Geometry check sheet. Reference: the model listing, model coordinates, mm. Face numbers are marked on the shaded views. A direction names the side the tool comes from. Coordinates: 2 decimals unless noted, no trailing zeros. Write each loop counter-clockwise with the first axis right and the second up, starting at its lowest first coordinate (ties: lowest second). Pieces come first, ordered by that corner, then holes. Notation, with made-up numbers: (20.5, -30.5) -> (40.5, -30.5) arc R13 ccw to (40.5, -15.5) -> close; hole circle Ø6 at (-2.75, -34.5). An arc over 180 degrees is marked (long way). Answer in a Markdown table with one row per item. Add a question column.
1. Depth check by flat-ended pin: P1, Ø20.5, axis at y = -92.5, z = -40, coming from the +X side; P2, Ø10, axis at y = 48.5, z = 3.5, coming from the +X side; P3, Ø4, axis at x = -20.5, z = -41, coming from the +Y side. Enter the tip coordinate at first touch or a pass-through.
2. Cross-section at D-D on y = -37. Record the cut outline in (x, z).
3. Set-up check for the marked faces 1, 2, 3, 4 and 5: record each of +Z, -Z, +X, -X, +Y, -Y from which the full face is reachable in a straight line by a thin tool's end or side.
4. Cross-section at A-A on y = 65.5. Record the cut outline in (x, z).
5. Cross-section at B-B on z = -23. Record the cut outline in (x, y).
6. Scan lines: L1, parallel to Y at x = 13.5, z = -5; L2, parallel to Z at x = 7, y = 29.5; L3, parallel to Z at x = 75.5, y = 95. Record each from-to range of solid material in increasing order. Write a range as from..to.
7. Cross-section at C-C on x = -9. Record the cut outline in (y, z), and give its area (3 significant figures).
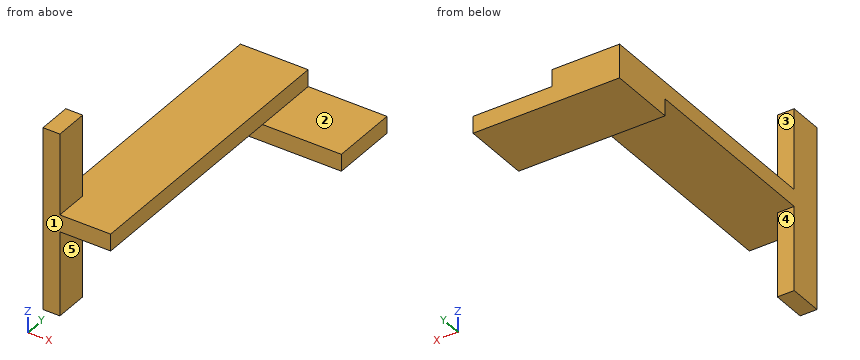
```python
from build123d import *

# Parameters (mm, degrees)
CROQUIS1_W              = 50.8
CROQUIS1_H              = 220
SALIENTE_EXTRUIR1_DEPTH = 12.7
CROQUIS2_W              = 110
CROQUIS2_H              = 50.8
SALIENTE_EXTRUIR2_DEPTH = 12.7
CROQUIS3_W              = 136.757374057
CROQUIS3_H              = 25.4
SALIENTE_EXTRUIR3_DEPTH = 12.7


with BuildPart() as part:
    # Croquis1 → Saliente-Extruir1 (new body)
    with BuildSketch(Plane.XY):
        Rectangle(CROQUIS1_W, CROQUIS1_H)
    extrude(amount=SALIENTE_EXTRUIR1_DEPTH)

    # Croquis2 → Saliente-Extruir2 (add)
    with BuildSketch(Plane(origin=(0, 0, 0), x_dir=(-1, 0, 0), z_dir=(0, 0, -1))):
        with Locations((-29.6, 84.6)):
            Rectangle(CROQUIS2_W, CROQUIS2_H)
    extrude(amount=SALIENTE_EXTRUIR2_DEPTH)

    # Croquis3 → Saliente-Extruir3 (add)
    with BuildSketch(Plane.ZY.offset(25.4)):
        with Locations((5.134235887, -97.3)):
            Rectangle(CROQUIS3_W, CROQUIS3_H)
    extrude(amount=-SALIENTE_EXTRUIR3_DEPTH)


solid = part.part
```
Results found:
| question | item | result |
|---|---|---|
| 1 | P1 | stops at x = -12.7 |
| 1 | P2 | stops at x = 25.4 |
| 1 | P3 | stops at y = -84.6 |
| 2 | outline | (-25.4, 0) -> (25.4, 0) -> (25.4, 12.7) -> (-25.4, 12.7) -> close |
| 3 | face 1 | +Z, -Z, +X, -X, -Y |
| 3 | face 2 | +Z, +X, +Y, -Y |
| 3 | face 3 | +Z, +X, -X, +Y |
| 3 | face 4 | -Z, +X, -X |
| 3 | face 5 | -Z, +X, -Y |
| 4 | outline | (-25.4, -12.7) -> (84.6, -12.7) -> (84.6, 0) -> (25.4, 0) -> (25.4, 12.7) -> (-25.4, 12.7) -> close |
| 5 | outline | (-25.4, -110) -> (-12.7, -110) -> (-12.7, -84.6) -> (-25.4, -84.6) -> close |
| 6 | L1 | y = 59.2..110 |
| 6 | L2 | z = 0..12.7 |
| 6 | L3 | z = -12.7..0 |
| 7 | outline | (-110, 0) -> (59.2, 0) -> (59.2, -12.7) -> (110, -12.7) -> (110, 12.7) -> (-110, 12.7) -> close |
| 7 | area | 3,440 mm^2 |
